from build123d import *

# Parameters (mm, degrees)
PAD016_DEPTH            = 10
SKETCH029_W             = 5
SKETCH029_H             = 5
POCKET013_DEPTH         = 10
CHAMFER_SIZE            = 5
BODY008_PLACEMENT_ANGLE = 70


with BuildPart() as part:
    # Sketch030 → Pad016 (new body)
    with BuildSketch(Plane.YZ):
        Polygon((0, 0), (47.88282, 131.556967), (117.88282, 131.556967), (117.88282, 10), (140, 10), (140, 0), align=None)
        Polygon((57.88282, 121.556967), (17.279405, 10), (107.88282, 10), (107.88282, 121.556967), align=None, mode=Mode.SUBTRACT)
    extrude(amount=PAD016_DEPTH)

    # Sketch029 → Pocket013 (cut)
    with BuildSketch(Plane.YZ):
        with Locations((112.5, 5)):
            Rectangle(SKETCH029_W, SKETCH029_H)
        with Locations((9.5, 5)):
            Rectangle(SKETCH029_W, SKETCH029_H)
        with Locations((52.5, 126.56)):
            Rectangle(SKETCH029_W, SKETCH029_H)
        with Locations((112.5, 126.56)):
            Rectangle(SKETCH029_W, SKETCH029_H)
        with Locations((52.5, 5)):
            Rectangle(SKETCH029_W, SKETCH029_H)
        with Locations((112.5, 65)):
            Rectangle(SKETCH029_W, SKETCH029_H)
    extrude(amount=POCKET013_DEPTH, mode=Mode.SUBTRACT)

    # Chamfer
    chamfer_edges = [part.edges().sort_by_distance(p)[0] for p in [
        (5, 117.88282, 10),
        (5, 107.88282, 10),
        (5, 107.88282, 121.556967),
        (5, 17.279405, 10),
    ]]
    chamfer(chamfer_edges, length=CHAMFER_SIZE)


with BuildPart() as part_1:
    # Body008 placement: moved
    add(part.part.moved(Location((-24, -19.731529, -6.864937))).rotate(Axis((-24, -19.731529, -6.864937), (-1, 0, 0)), BODY008_PLACEMENT_ANGLE))


solid = part_1.part
Model file for the job. Use its own axes, mm. A direction names the side the tool comes from. Coordinates: 2 decimals unless noted, no trailing zeros. Order: outer loops, then holes, each group sorted by start corner. A loop starts at its lowest first (then second) coordinate and runs counter-clockwise, first axis right, second up. Notation, with made-up numbers: (-26.75, -16.5) -> (-13.75, -16.5) arc R18 ccw to (-13.75, -4.5) -> close; hole circle Ø9 at (71.5, 86.25). An arc over 180 degrees is marked (long way). Return JSON: item names as keys, results as strings. Group by question number.
Item 1: Flat gauge pins, fed straight in: P1, Ø6, axis at x = -18.5, z = -104, coming from the -Y side; P2, Ø3, axis at x = -17.5, y = 75.5, coming from the -Z side; P3, Ø2, axis at x = -18.5, z = -114, coming from the +Y side. Where does each tip first touch, or does it go through?
Item 2: Wall check: line 1 along Y through (x, z) = (-21.5, -36.5); line 2 along Y through (x, z) = (-20.5, -24); line 3 along Z through (x, y) = (-22.25, 84.5). Give the ranges that are in metal, low to high. Write a range as [from, to].
Item 3: Saw through at C-C on x = -21. State how many separate pieces and enclosed holes the cut face has, then the cut area to 3 significant figures.
Item 4: Saw through at B-B on z = -33. Write the cut outline in (x, y), then the cut area to 3 significant figures.
Item 5: Pull direction Z, two halves, no side cores. Call faces 3 (the flat face through (-19.07, 122.095, -41.121)), 4 (the flat face through (-19, 49, -6.865)): pulls with the +Z half, pulls with the -Z half, needs draft (parallel to the pull), parting line crosses it, or undercut.
Item 6: Saw through at A-A on y = 18. Write the cut outline in (x, z), then the cut area to 3 significant figures.
Item 7: Tool access for faces 1 (the flat face through (-19.07, 34.58, -126.85)), 2 (the flat face through (-19.07, 138.495, -71.655)): list every direction of +Z, -Z, +X, -X, +Y, -Y with a clear straight run to the whole face (end or side of a thin tool).
Values found:
{
 "1": {"P1": "stops at y = 14.53", "P2": "stops at z = -98.2", "P3": "stops at y = 34.45"},
 "2": {"line 1": "y = [-8.95, 1.7], [120.41, 131.05]", "line 2": "y = [-13.49, -2.45], [115.86, 126.51]", "line 3": "z = [-94.38, -83.73], [-19.68, -6.86]"},
 "3": {"separate pieces": "1", "enclosed holes": "7", "area": "4,640 mm2"},
 "4": {"outline": "(-24, -10.22) -> (-14, -10.22) -> (-14, 0.42) -> (-24, 0.42) -> close; (-24, 119.14) -> (-14, 119.14) -> (-14, 129.78) -> (-24, 129.78) -> close", "area": "213 mm2"},
 "5": {"face 3": "undercut", "face 4": "pulls with the +Z half"},
 "6": {"outline": "(-24, -110.53) -> (-14, -110.53) -> (-14, -81.29) -> (-24, -81.29) -> close; (-24, -19.68) -> (-14, -19.68) -> (-14, -6.86) -> (-24, -6.86) -> close", "area": "421 mm2"},
 "7": {"face 1": "+X, -X, +Y", "face 2": "+X, -X"}
}
